Can you work these out from the model? Positions are in its coordinate system, mm. A direction names the side the tool comes from. Give positions to 0.01 mm unless a question says otherwise; leave off trailing zeros. Order: outer loops, then holes, each group sorted by start corner. A loop starts at its lowest first (then second) coordinate and runs counter-clockwise, first axis right, second up. Notation, with made-up numbers: (-18, -5.5) -> (24, -5.5) arc R26 cw to (24, 13.5) -> close; hole circle Ø9 at (13, -32.5). An arc over 180 degrees is marked (long way). Answer as a JSON object with one key per item and string values.
```python
from build123d import *

# Parameters (mm, degrees)
F0_R          = 8.5
F1_DEPTH      = 4
F2_R          = 5
F3_DEPTH      = 100
F5_DEPTH      = 25
F5_DEPTH_BACK = 25


with BuildPart() as f1:
    # F0 (on Top) → F1 (new body)
    with BuildSketch(Plane.XY):
        Circle(F0_R)
    extrude(amount=F1_DEPTH)

    # F2 (on Top) → F3 (join)
    with BuildSketch(Plane.XY):
        Circle(F2_R)
    extrude(amount=F3_DEPTH)

    # F4 (on Right) → F5 (cut, two sides)
    with BuildSketch(Plane.YZ) as f5_sk:
        Polygon((0, 101), (-5, 101), (-5, 96), align=None)
    extrude(amount=F5_DEPTH, mode=Mode.SUBTRACT)
    extrude(f5_sk.sketch, amount=-F5_DEPTH_BACK, mode=Mode.SUBTRACT)


solid = f1.part
```
1. If we section it at D-D on y = 7.25: Please give me the cut outline in (x, z), then the cut area to 3 significant figures.
Worked answers:
{"outline": "(-4.44, 0) -> (4.44, 0) -> (4.44, 4) -> (-4.44, 4) -> close", "area": "35.5 mm²"}
2. If we section it at C-C on z = 94.5: Please give me the cut outline in (x, y), then the cut area to 3 significant figures.
Worked answers:
{"outline": "circle Ø10 at (0, 0)", "area": "78.5 mm²"}
3. Please list where these lines run through material, in increasing order: L1, parallel to Z at x = 3.5, y = 7.5; L2, parallel to Y at x = 0, z = 29; L3, parallel to X at y = 2.75, z = 50.
Worked answers:
{"L1": "0 to 4", "L2": "-5 to 5", "L3": "-4.18 to 4.18"}
4. If we section it at B-B on x = 0: Please give me the cut outline in (y, z), then the cut area to 3 significant figures.
Worked answers:
{"outline": "(-8.5, 0) -> (8.5, 0) -> (8.5, 4) -> (5, 4) -> (5, 100) -> (-1, 100) -> (-5, 96) -> (-5, 4) -> (-8.5, 4) -> close", "area": "1,020 mm²"}
5. Will these pins go through, and if not, where does the flat tip stop? pin 1 Ø8 at (y, z) = (0.5, 24) entering from -X; pin 2 Ø10 at (y, z) = (-3.5, 90) entering from +X; pin 3 Ø1 at (y, z) = (-3, 62) entering from -X.
Worked answers:
{"pin 1": "x = -5", "pin 2": "x = 5", "pin 3": "x = -4.33"}
6. For faces 1 (the face through (0, 1, 100)), 2 (the face through (4, -4, 4)), which set-ups out of +Z, -Z, +X, -X, +Y, -Y let a thin tool reach every point of the face, with its end or its side?
Worked answers:
{"face 1": "+Z, +X, -X, +Y, -Y", "face 2": "+Z"}
7. If we section it at A-A on y = 0: Please give me the cut outline in (x, z).
Worked answers:
{"outline": "(-8.5, 0) -> (8.5, 0) -> (8.5, 4) -> (5, 4) -> (5, 100) -> (-5, 100) -> (-5, 4) -> (-8.5, 4) -> close"}
